from build123d import *

# Parameters (mm, degrees)
SKETCH009_R      = 0.5
EXTRUDE011_DEPTH = 8
SKETCH010_R      = 0.95
EXTRUDE010_DEPTH = 0.8
SKETCH008_W      = 96
SKETCH008_H      = 82
EXTRUDE009_DEPTH = 2
FILLET004_R      = 1
SKETCH007_W      = 92
SKETCH007_H      = 78
SKETCH007_W_2    = 88
SKETCH007_H_2    = 74
EXTRUDE008_DEPTH = 3


with BuildPart() as extrude011:
    # Sketch009 (on Face5 of Fusion002) → Extrude011 (new body)
    with BuildSketch(Plane.XY.offset(12)):
        with Locations((24.37, 40)):
            Circle(SKETCH009_R)
        with Locations((0, -40)):
            Circle(SKETCH009_R)
        with Locations((47, -40)):
            Circle(SKETCH009_R)
        with Locations((-47, -40)):
            Circle(SKETCH009_R)
        with Locations((-47, 40)):
            Circle(SKETCH009_R)
        with Locations((47, 40)):
            Circle(SKETCH009_R)
    extrude(amount=-EXTRUDE011_DEPTH)


with BuildPart() as fusion004:
    # Sketch010 (on Face5 of Fusion002) → Extrude010 (new body)
    with BuildSketch(Plane.XY.offset(12)):
        with Locations((24.37, 40)):
            Circle(SKETCH010_R)
        with Locations((0, -40)):
            Circle(SKETCH010_R)
        with Locations((47, -40)):
            Circle(SKETCH010_R)
        with Locations((-47, -40)):
            Circle(SKETCH010_R)
        with Locations((-47, 40)):
            Circle(SKETCH010_R)
        with Locations((47, 40)):
            Circle(SKETCH010_R)
    extrude(amount=-EXTRUDE010_DEPTH)

    # Fusion004: union Extrude011
    add(extrude011.part)


with BuildPart() as fillet004:
    # Sketch008 (on Face5 of Fusion001) → Extrude009 (new body)
    with BuildSketch(Plane.XY.offset(10)):
        Rectangle(SKETCH008_W, SKETCH008_H)
    extrude(amount=EXTRUDE009_DEPTH)

    # Fillet004
    fillet004_edges = [fillet004.edges().sort_by_distance(p)[0] for p in [
        (-48, 41, 11),
        (48, 41, 11),
        (48, -41, 11),
        (-48, -41, 11),
    ]]
    fillet(fillet004_edges, radius=FILLET004_R)


with BuildPart() as under001:
    # Sketch007 (on Face5 of Fusion001) → Extrude008 (new body)
    with BuildSketch(Plane.XY.offset(10)):
        Rectangle(SKETCH007_W, SKETCH007_H)
        Rectangle(SKETCH007_W_2, SKETCH007_H_2, mode=Mode.SUBTRACT)
    extrude(amount=-EXTRUDE008_DEPTH)

    # Fusion002: union Fillet004
    add(fillet004.part)

    # Cut004: cut Fusion004
    add(fusion004.part, mode=Mode.SUBTRACT)


solid = under001.part
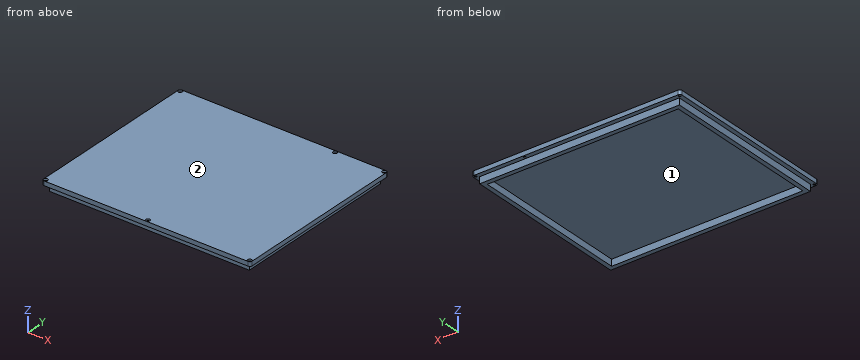
Input: part model. Units: mm. Frame: model coordinates. Face numbers are marked on the shaded views. Coordinates: 2 decimals unless noted, no trailing zeros. Write each loop counter-clockwise with the first axis right and the second up, starting at its lowest first coordinate (ties: lowest second). Pieces come first, ordered by that corner, then holes. Notation, with made-up numbers: M -21.75,74 L 23.25,74 A19 ccw 23.25,81 Z; hole C 84,62 d3. An arc over 180 degrees is marked long. Answer as a JSON object with one key per item and string values. Group by question number.
(1) Section B-B on x = 35.5. Output: boundary loops of the cut face in (y, z), plus the area to 3 significant figures.
(2) Section C-C on z = 8.25. Output: boundary loops of the cut face in (x, y).
(3) Contact query for flat-ended pins moving along their axis: P1, Ø1.5, axis at x = -5, z = 8, coming from the -Y side; P2, Ø1.5, axis at x = 47, y = -40, coming from the +Z side; P3, Ø1.5, axis at x = 3, z = 9, coming from the +Y side. Output: stop coordinate, or through.
(4) Ray query, line 1 along Y through (x, z) = (-47, 10.5); line 2 along X through (y, z) = (-40, 10.3); line 3 along X through (y, z) = (-6.5, 8.05). Return the intervals inside material, ascending. Write a range as [from, to].
(5) Section A-A on y = -22.5. Output: boundary loops of the cut face in (x, z), plus the area to 3 significant figures.
(6) Mould query, pull axis X, two halves, no side actions, for the marked faces 1 and 2. Classes: pulls with the +X half, pulls with the -X half, needs draft (parallel to the pull), parting line crosses it, or undercut.
Result set:
{
 "1": {"outline": "M -41,10 L -39,10 L -39,7 L -37,7 L -37,10 L 37,10 L 37,7 L 39,7 L 39,10 L 41,10 L 41,12 L -41,12 Z", "area": "176 mm2"},
 "2": {"outline": "M -46,-39 L 46,-39 L 46,39 L -46,39 Z; hole M -44,-37 L 44,-37 L 44,37 L -44,37 Z"},
 "3": {"P1": "stops at y = -39", "P2": "stops at z = 11.2", "P3": "stops at y = 39"},
 "4": {"line 1": "y = [-41, -40.5], [-39.5, 39.5], [40.5, 41]", "line 2": "x = [-48, -47.5], [-46.5, -0.5], [0.5, 46.5], [47.5, 48]", "line 3": "x = [-46, -44], [44, 46]"},
 "5": {"outline": "M -48,10 L -46,10 L -46,7 L -44,7 L -44,10 L 44,10 L 44,7 L 46,7 L 46,10 L 48,10 L 48,12 L -48,12 Z", "area": "204 mm2"},
 "6": {"face 1": "undercut", "face 2": "needs draft"}
}
